Build history of the part. All positions in model axes, mm. Round coordinates to 2 decimals unless told otherwise and drop trailing zeros. Write each loop counter-clockwise with the first axis right and the second up, starting at its lowest first coordinate (ties: lowest second). Pieces come first, ordered by that corner, then holes. Notation, with made-up numbers: (-14, 6.25) -> (10, 6.25) arc R17 cw to (10, 21.25) -> close; hole circle Ø2 at (-36.5, 77). An arc over 180 degrees is marked (long way). Return JSON: item names as keys, results as strings.
Autodesk Inventor part; units mm, degrees
ref_plane "YZ Plane" through (0, 0, 0) normal (1, 0, 0) x (0, 1, 0)
ref_plane "XZ Plane" through (0, 0, 0) normal (0, 1, 0) x (-1, 0, 0)
ref_plane "XY Plane" through (0, 0, 0) normal (0, 0, 1) x (1, 0, 0)
sketch "Sketch1" plane through (0, 0, 0) normal (0, 1, 0) x (-1, 0, 0)
  line L0 (-48, 0) -> (-48, 45)
  line L1 (-48, 45) -> (0, 45)
  line L2 (0, 45) -> (0, 0)
  line L3 (-6, 0) -> (-6, -85)
  line L4 (-6, -85) -> (-42, -85)
  line L5 (-42, -85) -> (-42, 0)
  line L6 (-24, 45) -> (-24, 29)
  circle A0 centre (-24, 25) radius 4
  line L7 (0, 0) -> (-6, 0)
  line L8 (-42, 0) -> (-48, 0)
  dimension "d8" = 8
  dimension "d0" = 48
  dimension "d1" = 45
  dimension "d2" = 36
  dimension "d3" = 85
  dimension "d6" = 16
  dimension "d7" = 6
extrude "Extrusion1" add sketch "Sketch1" along normal blind 1
properties part number "PendulumBackplate"
Q1. Pin check, flat tips, straight feed: pin 1 Ø3 at (x, z) = (36, -10) entering from -Y; pin 2 Ø6.5 at (x, z) = (24, 25) entering from -Y; pin 3 Ø0.5 at (y, z) = (0.5, -43) entering from -X. Stop position of each tip, or through.
Verdict:
{"pin 1": "stops at y = 0", "pin 2": "passes through", "pin 3": "stops at x = 6"}
Q2. Saw through at C-C on y = 0.5. List the corners of the cut face in (x, z).
Verdict:
{"outline": "(0, 0) -> (6, 0) -> (6, -85) -> (42, -85) -> (42, 0) -> (48, 0) -> (48, 45) -> (0, 45) -> close; hole circle Ø8 at (24, 25)"}
Q3. Saw through at B-B on x = 24. List the corners of the cut face in (y, z).
Verdict:
{"outline": "(0, -85) -> (1, -85) -> (1, 21) -> (0, 21) -> close; (0, 29) -> (1, 29) -> (1, 45) -> (0, 45) -> close"}
Q4. Two-plate mould, pull along X, no slides. Class faces 1 (the cylindrical face through (26.95, 0.49, 22.3)), 2 (the flat face through (24, 0, -19)): +X half, -X half, draft (parallel to the pull), parting line (faces both ways), or undercut.
Verdict:
{"face 1": "undercut", "face 2": "draft"}
Q5. Wall check: L1, parallel to X at y = 0.25, z = 25; L2, parallel to Z at x = 24, y = 0.2; L3, parallel to X at y = 0.7, z = -53.5. Give the ranges that are in metal, low to high.
Verdict:
{"L1": "x = 0 to 20, 28 to 48", "L2": "z = -85 to 21, 29 to 45", "L3": "x = 6 to 42"}
Q6. Saw through at A-A on z = 25. List the corners of the cut face in (x, y).
Verdict:
{"outline": "(0, 0) -> (20, 0) -> (20, 1) -> (0, 1) -> close; (28, 0) -> (48, 0) -> (48, 1) -> (28, 1) -> close"}
Q7. Saw through at D-D on x = 4. List the corners of the cut face in (y, z).
Verdict:
{"outline": "(0, 0) -> (1, 0) -> (1, 45) -> (0, 45) -> close"}
